Check sheet for the modelled part. Datum: model origin and axes. Units: mm. Face numbers are marked on the shaded views. A direction names the side the tool comes from. Coordinates: 2 decimals unless noted, no trailing zeros. Order: outer loops, then holes, each group sorted by start corner. A loop starts at its lowest first (then second) coordinate and runs counter-clockwise, first axis right, second up.
Autodesk Inventor part; units mm, degrees
ref_plane "YZ Plane" through (0, 0, 0) normal (1, 0, 0) x (0, 1, 0)
ref_plane "XZ Plane" through (0, 0, 0) normal (0, 1, 0) x (-1, 0, 0)
ref_plane "XY Plane" through (0, 0, 0) normal (0, 0, 1) x (1, 0, 0)
sketch "Sketch1" plane through (0, 0, 0) normal (0, 0, 1) x (1, 0, 0)
  line L0 (-3.81, -8.89) -> (3.81, -8.89)
  line L1 (3.81, -8.89) -> (3.81, 8.89)
  line L2 (3.81, 8.89) -> (-3.81, 8.89)
  line L3 (-3.81, 8.89) -> (-3.81, -8.89)
  line L4 (-3.81, -8.89) -> (3.81, 8.89) construction
  line L5 (3.81, -8.89) -> (-3.81, 8.89) construction
  line L6 (-3.048, 3.048) -> (3.048, 3.048)
  line L7 (3.048, 3.048) -> (3.048, 8.128)
  line L8 (3.048, 8.128) -> (-3.048, 8.128)
  line L9 (-3.048, 8.128) -> (-3.048, 3.048)
  line L10 (-3.048, 3.048) -> (3.048, 8.128) construction
  line L11 (3.048, 3.048) -> (-3.048, 8.128) construction
  circle A0 centre (0, -3.302) radius 2.794
  point P0 (0, 0)
  point P1 (0, 5.588)
  dimension "d0" = 7.62
  dimension "d1" = 17.78
  dimension "d2" = 0.762
  dimension "d3" = 0.762
  dimension "d4" = 0.762
  dimension "d5" = 5.08
  dimension "d6" = 5.588
  dimension "d7" = 5.588
extrude "Extrusion1" add sketch "Sketch1" along normal blind 1.778 contours L3 L2 L1 L0 | L9 L8 L7 L6 | A0
fillet "Fillet1" radius 0.762 4 edges at (3.81, 0, 0) (3.81, 0, 1.778) (-3.81, 0, 1.778) (-3.81, 0, 0)
extrude "Extrusion2" cut sketch "Sketch1" along normal blind 0.0254 contours L9 L8 L7 L6
fillet "Fillet2" radius 0.254 4 edges at (3.048, 8.128, 0.0127) (-3.048, 8.128, 0.0127) (3.048, 3.048, 0.0127) (-3.048, 3.048, 0.0127)
sketch "Sketch2" plane through (0, 0, 0) normal (0, 0, -1) x (-1, 0, 0)
  circle A0 centre (0, -3.302) radius 1.016
  circle A1 centre (0, -3.302) radius 2.794
  point P0 (0, 0)
  dimension "d14" = 2.032
extrude "Extrusion3" add sketch "Sketch2" along normal blind 0.0508
fillet "Fillet3" radius 0.0254 2 edges at (1.016, -3.302, -0.0508) (2.794, -3.302, -0.0508)
sketch "Sketch3" plane through (0, -3.302, -0.0508) normal (0, 0, -1) x (-1, 0, 0)
  line L0 (-0.9463, 2.473) -> (1.05, 2.473) construction
  line L1 (1.05, 2.473) -> (1.05, 1.9797) construction
  line L2 (1.05, 1.9797) -> (-0.9463, 1.9797) construction
  line L3 (-0.9463, 1.9797) -> (-0.9463, 2.473) construction
  line L4 (-2.6797, -0.254) -> (-2.6035, -0.254)
  line L5 (-2.6035, -0.254) -> (-2.6035, 0.254)
  line L6 (-2.6035, 0.254) -> (-2.6797, 0.254)
  line L7 (-2.6797, 0.254) -> (-2.6797, -0.254)
  line L8 (-2.6797, -0.254) -> (-2.6035, 0.254) construction
  line L9 (-2.6035, -0.254) -> (-2.6797, 0.254) construction
  line L10 (0, 0) -> (0, 3.302) construction
  line L11 (-2.5273, 0) -> (-2.2733, 0.254)
  line L12 (-2.2733, 0.254) -> (-2.2733, -0.254)
  line L13 (-2.2733, -0.254) -> (-2.5273, 0)
  line L14 (-2.1971, 0) -> (-1.9431, 0.254)
  line L15 (-1.9431, 0.254) -> (-1.9431, -0.254)
  line L16 (-3.048, 12.192) -> (-3.048, -5.588)
  line L17 (-1.9431, -0.254) -> (-2.1971, 0)
  line L18 (2.6797, -0.254) -> (2.6035, -0.254)
  line L19 (2.6035, -0.254) -> (2.6035, 0.254)
  line L20 (2.6035, 0.254) -> (2.6797, 0.254)
  line L21 (2.6797, 0.254) -> (2.6797, -0.254)
  line L22 (2.6797, -0.254) -> (2.6035, 0.254) construction
  line L23 (2.6035, -0.254) -> (2.6797, 0.254) construction
  line L24 (2.5273, 0) -> (2.2733, 0.254)
  line L25 (2.2733, 0.254) -> (2.2733, -0.254)
  line L26 (2.2733, -0.254) -> (2.5273, 0)
  line L27 (2.1971, 0) -> (1.9431, 0.254)
  line L28 (1.9431, 0.254) -> (1.9431, -0.254)
  line L29 (1.9431, -0.254) -> (2.1971, 0)
  line L30 (-0.2936, -2.0988) -> (-0.0396, -2.3528)
  line L31 (-0.0396, -2.3528) -> (-0.2936, -2.6068)
  line L32 (-0.2936, -2.6068) -> (-0.2936, -2.0988)
  line L33 (0.0874, -2.6138) -> (0.1636, -2.6138)
  line L34 (0.1636, -2.6138) -> (0.1636, -2.0919)
  line L35 (0.1636, -2.0919) -> (0.0874, -2.0919)
  line L36 (0.0874, -2.0919) -> (0.0874, -2.6138)
  line L37 (0.0874, -2.6138) -> (0.1636, -2.0919) construction
  line L38 (0.1636, -2.6138) -> (0.0874, -2.0919) construction
  line L39 (0.2398, -2.6138) -> (0.316, -2.6138)
  line L40 (0.316, -2.6138) -> (0.316, -2.0919)
  line L41 (0.316, -2.0919) -> (0.2398, -2.0919)
  line L42 (0.2398, -2.0919) -> (0.2398, -2.6138)
  line L43 (0.2398, -2.6138) -> (0.316, -2.0919) construction
  line L44 (0.316, -2.6138) -> (0.2398, -2.0919) construction
  line L45 (-2.6416, 0) -> (0, 0) construction
  line L46 (-0.903, 2.092) -> (-0.903, 2.473)
  line L47 (-0.903, 2.473) -> (-0.8197, 2.473)
  line L48 (-0.8197, 2.473) -> (-0.7203, 2.2033)
  spline S0 degree 2 poles (-0.7203, 2.2033) (-0.7067, 2.1655) (-0.7003, 2.1469) knots 0 0 0 1 1 1
  spline S1 degree 2 poles (-0.7003, 2.1469) (-0.6933, 2.1675) (-0.6782, 2.2079) knots 0 0 0 1 1 1
  line L49 (-0.6782, 2.2079) -> (-0.5775, 2.473)
  line L50 (-0.5775, 2.473) -> (-0.5031, 2.473)
  line L51 (-0.5031, 2.473) -> (-0.5031, 2.092)
  line L52 (-0.5031, 2.092) -> (-0.5566, 2.092)
  line L53 (-0.5566, 2.092) -> (-0.5566, 2.4109)
  line L54 (-0.5566, 2.4109) -> (-0.6785, 2.092)
  line L55 (-0.6785, 2.092) -> (-0.7285, 2.092)
  line L56 (-0.7285, 2.092) -> (-0.8496, 2.4164)
  line L57 (-0.8496, 2.4164) -> (-0.8496, 2.092)
  line L58 (-0.8496, 2.092) -> (-0.903, 2.092)
  line L59 (-0.4128, 2.092) -> (-0.4128, 2.473)
  line L60 (-0.4128, 2.473) -> (-0.1099, 2.473)
  line L61 (-0.1099, 2.473) -> (-0.1099, 2.428)
  line L62 (-0.1099, 2.428) -> (-0.3573, 2.428)
  line L63 (-0.3573, 2.428) -> (-0.3573, 2.3116)
  line L64 (-0.3573, 2.3116) -> (-0.1256, 2.3116)
  line L65 (-0.1256, 2.3116) -> (-0.1256, 2.2666)
  line L66 (-0.1256, 2.2666) -> (-0.3573, 2.2666)
  line L67 (-0.3573, 2.2666) -> (-0.3573, 2.137)
  line L68 (-0.3573, 2.137) -> (-0.1003, 2.137)
  line L69 (-0.1003, 2.137) -> (-0.1003, 2.092)
  line L70 (-0.1003, 2.092) -> (-0.4128, 2.092)
  line L71 (-0.0246, 2.092) -> (-0.0246, 2.473)
  line L72 (-0.0246, 2.473) -> (0.0324, 2.473)
  line L73 (0.0324, 2.473) -> (0.2522, 2.1739)
  line L74 (0.2522, 2.1739) -> (0.2522, 2.473)
  line L75 (0.2522, 2.473) -> (0.3053, 2.473)
  line L76 (0.3053, 2.473) -> (0.3053, 2.092)
  line L77 (0.3053, 2.092) -> (0.2484, 2.092)
  line L78 (0.2484, 2.092) -> (0.0286, 2.3911)
  line L79 (0.0286, 2.3911) -> (0.0286, 2.092)
  line L80 (0.0286, 2.092) -> (-0.0246, 2.092)
  line L81 (0.673, 2.473) -> (0.7284, 2.473)
  line L82 (0.7284, 2.473) -> (0.7284, 2.2529)
  spline S2 degree 2 poles (0.7284, 2.2529) (0.7284, 2.1954) (0.7, 2.128) (0.6254, 2.0856) (0.5647, 2.0856) knots 0 0 0 1 2 3 3 3
  spline S3 degree 2 poles (0.5647, 2.0856) (0.506, 2.0856) (0.4311, 2.1225) (0.3991, 2.1925) (0.3991, 2.2529) knots 0 0 0 1 2 3 3 3
  line L83 (0.3991, 2.2529) -> (0.3991, 2.473)
  line L84 (0.3991, 2.473) -> (0.4546, 2.473)
  line L85 (0.4546, 2.473) -> (0.4546, 2.2532)
  spline S4 degree 2 poles (0.4546, 2.2532) (0.4546, 2.2038) (0.4749, 2.1568) (0.5243, 2.1312) (0.56, 2.1312) knots 0 0 0 1 2 3 3 3
  spline S5 degree 2 poles (0.56, 2.1312) (0.621, 2.1312) (0.673, 2.1818) (0.673, 2.2532) knots 0 0 0 1 2 2 2
  line L86 (0.673, 2.2532) -> (0.673, 2.473)
  point P0 (2.6416, 0)
  point P1 (0.1255, -2.3528)
  point P2 (0.2779, -2.3528)
  dimension "d18" = 0.254
  dimension "d19" = 0.254
  dimension "d22" = 0.508
  dimension "d23" = 0.254
  dimension "d24" = 3.302
  dimension "d25" = 2.6416
  dimension "d26" = 0.0762
  dimension "d27" = 0.0762
  dimension "d28" = 0.0762
  dimension "d29" = 0.254
  dimension "d30" = 0.508
  dimension "d31" = 0.254
  dimension "d32" = 0.127
  dimension "d33" = 0.0762
  dimension "d34" = 0.0762
extrude "Extrusion4" cut sketch "Sketch3" against normal blind 0.0127
properties part number "iPod Nano"
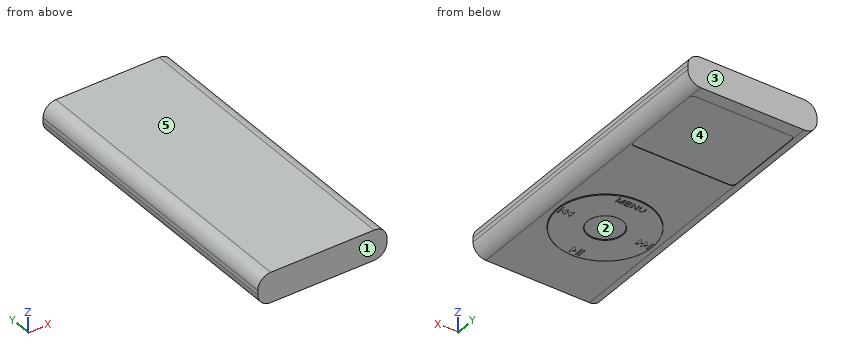
(1) Tool access check on the marked faces 1 and 2. Record the directions out of +Z, -Z, +X, -X, +Y, -Y that give a thin tool (end or side, any length) a straight path to the whole face; none if there is none.
Filled in:
face 1: +Z, -Z, +X, -X, -Y
face 2: -Z
(2) Cross-section at D-D (z = 1.4). Enter the section's corners in (x, y), and give its area (3 significant figures).
Filled in:
outline: (-3.71, -8.89) - (3.71, -8.89) - (3.71, 8.89) - (-3.71, 8.89) - close
area: 132 mm2
(3) Thickness scan on probe 1 along Z at (x, y) = (-3, -1); probe 2 along X at (y, z) = (3.25, 1.45); probe 3 along X at (y, z) = (-5.5, 0.15). Record the ranges inside material, lowest first.
Filled in:
probe 1: z = 0 to 1.78
probe 2: x = -3.67 to 3.67
probe 3: x = -3.5 to 3.5
(4) Cross-section at C-C (x = -3.5). Enter the section's corners in (y, z).
Filled in:
outline: (-8.89, 0.15) - (8.89, 0.15) - (8.89, 1.63) - (-8.89, 1.63) - close
(5) Cross-section at B-B (y = 1.75). Enter the section's corners in (x, z), and give its area (3 significant figures).
Filled in:
outline: (-3.81, 0.76) arc R0.76 ccw to (-3.05, 0) - (3.05, 0) arc R0.76 ccw to (3.81, 0.76) - (3.81, 1.02) arc R0.76 ccw to (3.05, 1.78) - (-3.05, 1.78) arc R0.76 ccw to (-3.81, 1.02) - close
area: 13.0 mm2
(6) Release check for a two-part mould opening along Y. For the marked faces 3, 4 and 5 record: +Y half, -Y half, draft (parallel to the pull), parting line (faces both ways), or undercut.
Filled in:
face 3: +Y half
face 4: undercut
face 5: draft
